Geometry: final body of the model. Coordinates: model frame, mm. Face numbers are marked on the shaded views. A direction names the side the tool comes from. Coordinates: 2 decimals unless noted, no trailing zeros. Order: outer loops, then holes, each group sorted by start corner. A loop starts at its lowest first (then second) coordinate and runs counter-clockwise, first axis right, second up. Notation, with made-up numbers: (17, 40.5) -> (48, 40.5) arc R21 cw to (48, 57.5) -> close; hole circle Ø2 at (-2.75, 15.5). An arc over 180 degrees is marked (long way). Use one line per item in the form item = value.
```python
from build123d import *

# Parameters (mm, degrees)
EXTRUDE_1_DEPTH = 8
CHAMFER_1_SIZE  = 2


with BuildPart() as part:
    # 草图1 → 旋转1 (revolve)
    with BuildSketch(Plane(origin=(0, 0, 0), x_dir=(1, 0, 0), z_dir=(0, 1, 0))):
        with BuildLine():
            Line((4, 0), (4, 8))
            Line((4, 8), (8, 8))
            Line((8, 8), (8, 31))
            Line((8, 31), (9.5, 31))
            Line((9.5, 31), (9.5, 70.5))
            Line((9.5, 70.5), (13, 70.5))
            Line((13, 70.5), (13, 75.5))
            ThreePointArc((13, 75.5), (6.519202405, 76.249631268), (0, 76.5))
            Line((0, 76.5), (0, -4))
            ThreePointArc((0, -4), (2.828427125, -2.828427125), (4, 0))
        make_face()
    revolve(axis=Axis((0, 0, 0), (0, 0, -1)))

    # 草图2 → 凸台-拉伸1 (add)
    with BuildSketch(Plane.XY.offset(-31)):
        Polygon((10.969655115, 0), (5.484827557, 9.5), (-5.484827557, 9.5), (-10.969655115, 0), (-5.484827557, -9.5), (5.484827557, -9.5), align=None)
    extrude(amount=-EXTRUDE_1_DEPTH)

    # 倒角1
    chamfer_1_edges = [part.edges().sort_by_distance(p)[0] for p in [
        (-8, 0, -8),
    ]]
    chamfer(chamfer_1_edges, length=CHAMFER_1_SIZE)


solid = part.part
```
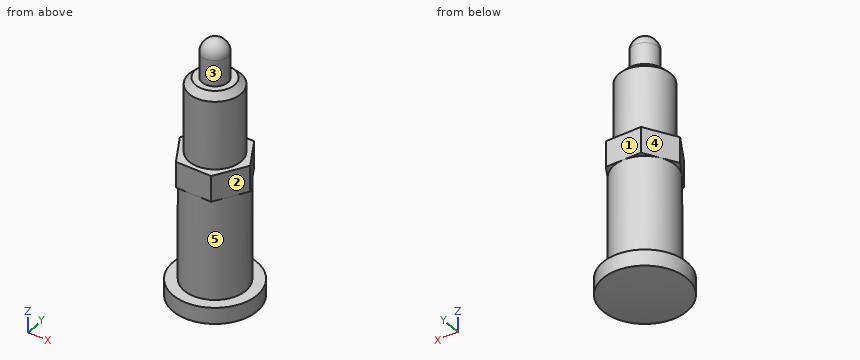
1) Section A-A, the plane z = -62.5. Output: boundary loops of the cut face in (x, y).
Results found:
outline = circle Ø19 at (0, 0)
2) Section C-C, the plane z = -14. Output: boundary loops of the cut face in (x, y), and give its area (3 significant figures).
Results found:
outline = circle Ø16 at (0, 0)
area = 201 mm2
3) Access query for the marked faces 1, 2 and 3. Directions: +Z, -Z, +X, -X, +Y, -Y. A direction counts if a zero-diameter tool reaches every point of the face in a straight line with its end or side. Return the directions, or none.
Results found:
face_1 = +Z, +X, -X, +Y
face_2 = +Z, +X, -Y
face_3 = +Z
4) Section B-B, the plane x = 11.75. Output: boundary loops of the cut face in (y, z), and give its area (3 significant figures).
Results found:
outline = (-5.56, -75.5) arc R84.18 ccw to (5.56, -75.5) -> (5.56, -70.5) -> (-5.56, -70.5) -> close
area = 57.0 mm2
5) Contact query for flat-ended pins moving along their axis: P1, Ø0.8, axis at x = 10, y = -1, coming from the -Z side; P2, Ø5, axis at y = 0.5, z = -32.5, coming from the +X side; P3, Ø1.5, axis at y = -7, z = -28, coming from the +X side. Output: stop coordinate, or through.
Results found:
P1 = -75.95
P2 = 10.97
P3 = 4.99
6) Material intervals for probe 1 along X at (y, z) = (3, -50); probe 2 along Z at (x, y) = (2, 11); probe 3 along Z at (x, y) = (11, -3.5), sorted ascending. Write a range as from..to.
Results found:
probe_1 = -9.01..9.01
probe_2 = -75.76..-70.5
probe_3 = -75.71..-70.5
7) Pull-direction query (Z, two-part tool) for the marked faces 4 and 5; classes: released by +Z, released by -Z, zero draft, split by the parting line, or undercut.
Results found:
face_4 = zero draft
face_5 = undercut
